Part model, mm, in its own coordinate system. Give positions to 0.01 mm unless a question says otherwise; leave off trailing zeros. Order: outer loops, then holes, each group sorted by start corner. A loop starts at its lowest first (then second) coordinate and runs counter-clockwise, first axis right, second up. Notation, with made-up numbers: (-17, -34.5) - (9, -34.5) arc R13 ccw to (9, -26.5) - close; hole circle Ø4 at (75.5, 33.5). An arc over 180 degrees is marked (long way). Use one line per item in the form item = value. Start each with the question number.
1. Band-saw the part on A-A, the plane y = 0. List the corners of the cut face in (x, z), plus the area to 3 significant figures.
2. Pin check, flat tip, straight feed: P1, Ø6, axis at x = 38.1, y = 0, coming from the -Z side. Stop position of the tip, or through.
3. Drill centre lines: line 1 (Y direction, x = 38.1, z = 13.5); line 2 (Y direction, x = 39.5, z = 9.75); line 3 (X direction, y = 25.4, z = 16.25). Where is each one in solid material? Low to high.
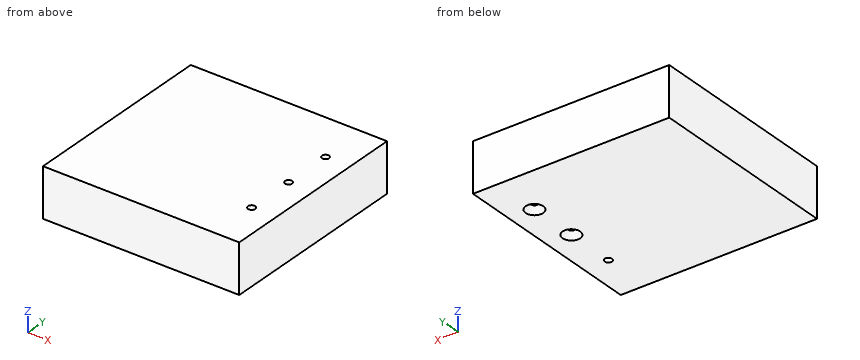
from build123d import *

# Parameters (mm, degrees)
F0_W           = 101.6
F0_H           = 101.6
F1_DEPTH       = 25.4
F2_D           = 3.7973
F3_D           = 3.6576
F3_CSINK_D     = 9.1186
F3_CSINK_ANGLE = 82


with BuildPart() as f1:
    # F0 (on Top) → F1 (new body)
    with BuildSketch(Plane.XY):
        Rectangle(F0_W, F0_H)
    extrude(amount=F1_DEPTH)

    # F2 (through all)
    with Locations(Plane(origin=(0, 0, 0), x_dir=(1, 0, 0), z_dir=(0, 0, -1))):
        with Locations((38.1, 25.4)):
            Hole(F2_D / 2)

    # F3 (through all)
    with Locations(Plane(origin=(0, 0, 0), x_dir=(1, 0, 0), z_dir=(0, 0, -1))):
        with Locations((38.1, 0), (38.1, -25.4)):
            CounterSinkHole(F3_D / 2, F3_CSINK_D / 2, counter_sink_angle=F3_CSINK_ANGLE)


solid = f1.part
From the geometry:
q1.outline = (-50.8, 0) - (33.54, 0) - (36.27, 3.14) - (36.27, 25.4) - (-50.8, 25.4) - close; (39.93, 3.14) - (42.66, 0) - (50.8, 0) - (50.8, 25.4) - (39.93, 25.4) - close
q1.area = 2,480 mm²
q2.P1 = 1.79
q3.line_1 = -50.8 to -27.3, -23.5 to -1.83, 1.83 to 23.57, 27.23 to 50.8
q3.line_2 = -50.8 to -26.68, -24.12 to -1.18, 1.18 to 24.22, 26.58 to 50.8
q3.line_3 = -50.8 to 36.27, 39.93 to 50.8
